Source: CAD feature listing. Evaluate the final solid. Frame: model axes, mm. A direction names the side the tool comes from. Give positions to 0.01 mm unless a question says otherwise; leave off trailing zeros. Order: outer loops, then holes, each group sorted by start corner. A loop starts at its lowest first (then second) coordinate and runs counter-clockwise, first axis right, second up.
from build123d import *

# Parameters (mm, degrees)
BOSS_EXTRUDE1_DEPTH = 15
CUT_EXTRUDE1_DEPTH  = 23.004565192
CUT_EXTRUDE2_DEPTH  = 23.004565192
SKETCH4_W           = 2.5
SKETCH4_H           = 2.5
SKETCH5_W           = 2.5
SKETCH5_H           = 2.5


with BuildPart() as part:
    # Sketch1 → Boss-Extrude1 (new body)
    with BuildSketch(Plane.XZ.offset(15)):
        with BuildLine():
            Line((-2.5, 14.272294466), (-2.5, 4.272294466))
            ThreePointArc((-2.5, 4.272294466), (0, -4.95), (2.5, 4.272294466))
            Line((2.5, 4.272294466), (2.5, 14.272294466))
            Line((2.5, 14.272294466), (-2.5, 14.272294466))
        make_face()
    extrude(amount=-BOSS_EXTRUDE1_DEPTH)

    # Sketch2 → Cut-Extrude1 (cut, through all)
    with BuildSketch(Plane(origin=(2.5, 0, 0), x_dir=(0, 0, -1), z_dir=(1, 0, 0))):
        with BuildLine():
            Line((-14.272294466, -15), (-9.272294466, -15))
            ThreePointArc((-9.272294466, -15), (-10.203329527, -13.83309751), (-11.437357975, -12.993060906))
            ThreePointArc((-11.437357975, -12.993060906), (-13.504629374, -11.148327894), (-14.272294466, -8.486121811))
            Line((-14.272294466, -8.486121811), (-14.272294466, -15))
        make_face()
    extrude(amount=-CUT_EXTRUDE1_DEPTH, mode=Mode.SUBTRACT)

    # Sketch3 → Cut-Extrude2 (cut, through all)
    with BuildSketch(Plane(origin=(2.5, 0, 0), x_dir=(0, 0, -1), z_dir=(1, 0, 0))):
        with BuildLine():
            Line((-9.272294466, 0), (-14.272294466, 0))
            Line((-14.272294466, 0), (-14.272294466, -6.513878189))
            ThreePointArc((-14.272294466, -6.513878189), (-13.504629374, -3.851672106), (-11.437357975, -2.006939094))
            ThreePointArc((-11.437357975, -2.006939094), (-10.203329527, -1.16690249), (-9.272294466, 0))
        make_face()
    extrude(amount=-CUT_EXTRUDE2_DEPTH, mode=Mode.SUBTRACT)

    # Sketch4 → Revolve1 (revolve)
    with BuildSketch(Plane(origin=(0, 0, 10.203329527), x_dir=(-1, 0, 0), z_dir=(0, 0, -1)), mode=Mode.PRIVATE) as revolve1_sk:
        with Locations((3.75, -6.25)):
            Rectangle(SKETCH4_W, SKETCH4_H)
    revolve(revolve1_sk.sketch.rotate(Axis((-2.5, -7.5, 10.203329527), (-1, 0, 0)), 270), axis=Axis((-2.5, -7.5, 10.203329527), (-1, 0, 0)))

    # Sketch5 → Revolve2 (revolve)
    with BuildSketch(Plane(origin=(0, 0, 10.203329527), x_dir=(-1, 0, 0), z_dir=(0, 0, -1)), mode=Mode.PRIVATE) as revolve2_sk:
        with Locations((-3.75, -6.25)):
            Rectangle(SKETCH5_W, SKETCH5_H)
    revolve(revolve2_sk.sketch.rotate(Axis((5, -7.5, 10.203329527), (-1, 0, 0)), 270), axis=Axis((5, -7.5, 10.203329527), (-1, 0, 0)))


solid = part.part
1) Section query B-B on y = -7.5. Output: boundary loops of the cut face in (x, z).
Checks:
outline: (-5, 7.7) - (-2.5, 7.7) - (-2.5, 4.27) arc R4.95 ccw (long way) to (2.5, 4.27) - (2.5, 7.7) - (5, 7.7) - (5, 12.7) - (2.5, 12.7) - (2.5, 14.27) - (-2.5, 14.27) - (-2.5, 12.7) - (-5, 12.7) - close
2) Section query A-A on x = 0. Output: boundary loops of the cut face in (y, z).
Checks:
outline: (-15, -4.95) - (0, -4.95) - (0, 9.27) arc R5 cw to (-2.01, 11.44) arc R5 ccw to (-6.51, 14.27) - (-8.49, 14.27) arc R5 ccw to (-12.99, 11.44) arc R5 cw to (-15, 9.27) - close
3) Reachability of faces 1 (the face through (-0.181, -7.605, -4.947)), 2 (the face through (-3.768, -9.718, 11.357)), 3 (the face through (2.5, -8, 7)) from +Z, -Z, +X, -X, +Y, -Y: full face, straight path, thin tool, end or side. Return the list, or none.
Checks:
face 1: +Y, -Y
face 2: -X
face 3: +X
4) Pull-direction query (Z, two-part tool) for faces 4 (the face through (0, 0, 2)), 5 (the face through (3.732, -9.718, 11.357)), 6 (the face through (0, -8, 14.272)); classes: +Z half, -Z half, draft (parallel to the pull), parting line (faces both ways), or undercut.
Checks:
face 4: draft
face 5: undercut
face 6: +Z half
5) Section query D-D on z = 13. Output: boundary loops of the cut face in (x, y), and give its area (3 significant figures).
Checks:
outline: (-2.5, -11.82) - (2.5, -11.82) - (2.5, -3.18) - (-2.5, -3.18) - close
area: 43.2 mm2
6) First-contact query: pin 1 Ø4 at (x, y) = (2.5, -4) entering from +Z; pin 2 Ø2 at (y, z) = (-5, 4.5) entering from +X; pin 3 Ø1.5 at (y, z) = (-12, 10.5) entering from +X. Flat tips, straight axial feed; report the tip coordinate or a pass-through.
Checks:
pin 1: stops at z = 14.25
pin 2: stops at x = 3.5
pin 3: stops at x = 2.5
7) Ray query, L1, parallel to X at y = -8, z = 5; L2, parallel to Z at x = -4, y = -9.25; L3, parallel to X at y = -13.5, z = -0.75. Return the intervals inside material, ascending.
Checks:
L1: x = -2.5 to 2.5
L2: z = -2.92 to 2.92, 8.42 to 11.99
L3: x = -4.89 to 4.89
8) Section query C-C on x = -4.5. Output: boundary loops of the cut face in (y, z).
Checks:
outline: (-15, -2.06) - (0, -2.06) - (0, 2.06) - (-15, 2.06) - close; circle Ø5 at (-7.5, 10.2)
